Here's how the part is built. I have some questions about the finished solid (model axes, mm). Round coordinates to 2 decimals unless told otherwise and drop trailing zeros. Order: outer loops, then holes, each group sorted by start corner. A loop starts at its lowest first (then second) coordinate and runs counter-clockwise, first axis right, second up.
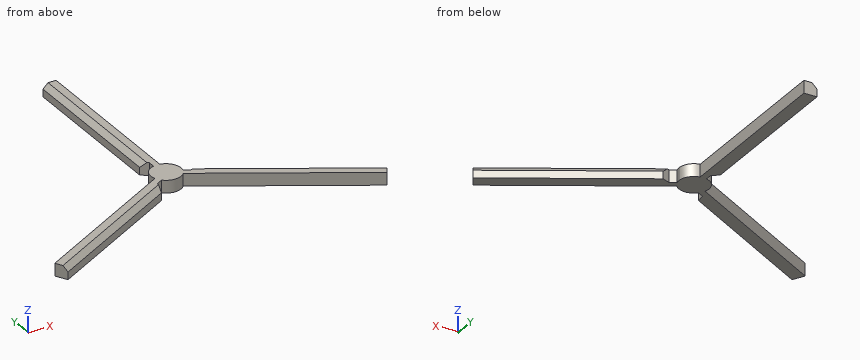
```python
from build123d import *

# Parameters (mm, degrees)
F1_DEPTH = 1.27
F2_SIZE  = 0.508


with BuildPart() as f1:
    # F0 (on Top) → F1 (new body)
    with BuildSketch(Plane.XY):
        with BuildLine():
            ThreePointArc((1.470624, -0.3998), (1.510597, -0.201674), (1.524, 0))
            ThreePointArc((1.524, 0), (1.166482, 0.980762), (0.261671, 1.501367))
            ThreePointArc((0.261671, 1.501367), (-0.065208, 1.522604), (-0.389075, 1.473498))
            ThreePointArc((-0.389075, 1.473498), (-1.351218, 0.70483), (-1.431058, -0.52407))
            ThreePointArc((-1.431058, -0.52407), (-1.28601, -0.817774), (-1.081549, -1.073698))
            ThreePointArc((-1.081549, -1.073698), (0.065208, -1.522604), (1.169387, -0.977297))
            ThreePointArc((1.169387, -0.977297), (1.351218, -0.70483), (1.470624, -0.3998))
        make_face()
        with BuildLine():
            ThreePointArc((-0.389075, 1.473498), (-0.065208, 1.522604), (0.261671, 1.501367))
            Line((0.261671, 1.501367), (0.261671, 19.281367))
            Line((0.261671, 19.281367), (-1.068548, 19.281367))
            Line((-1.068548, 19.281367), (-1.068548, 2.698131))
            Line((-1.068548, 2.698131), (-0.389075, 2.191366))
            Line((-0.389075, 2.191366), (-0.389075, 1.473498))
        make_face()
        with BuildLine():
            Line((2.092316, -0.758734), (1.470624, -0.3998))
            ThreePointArc((1.470624, -0.3998), (1.351218, -0.70483), (1.169387, -0.977297))
            Line((1.169387, -0.977297), (16.567319, -9.867297))
            Line((16.567319, -9.867297), (17.232428, -8.715294))
            Line((17.232428, -8.715294), (2.870924, -0.423675))
            Line((2.870924, -0.423675), (2.092316, -0.758734))
        make_face()
        with BuildLine():
            ThreePointArc((-1.081549, -1.073698), (-1.28601, -0.817774), (-1.431058, -0.52407))
            Line((-1.431058, -0.52407), (-16.82899, -9.41407))
            Line((-16.82899, -9.41407), (-16.16388, -10.566074))
            Line((-16.16388, -10.566074), (-1.802376, -2.274455))
            Line((-1.802376, -2.274455), (-1.703241, -1.432632))
            Line((-1.703241, -1.432632), (-1.081549, -1.073698))
        make_face()
    extrude(amount=F1_DEPTH)

    # F2
    f2_edges = [f1.edges().sort_by_distance(p)[0] for p in [
        (-1.068548, 10.989749, 1.27),
        (-8.983128, -6.420265, 1.27),
        (10.051676, -4.569485, 1.27),
    ]]
    chamfer(f2_edges, length=F2_SIZE)


solid = f1.part
```
1) If we section it at B-B (z = 0.2): Write out the boundary of the cut face in (x, y), plus the area to 3 significant figures.
2) If we section it at D-D (x = 11): Write out the boundary of the cut face in (y, z).
3) If we section it at A-A (y = -3.5): Write out the boundary of the cut face in (x, z).
4) I need wall thicknesses on line 1 (X direction, y = 13.5, z = 0.25); line 2 (X direction, y = -4.25, z = 0.35); line 3 (X direction, y = 7.5, z = 0.85). Which ranges of each line are inside material? Lowest first, please.
5) If we section it at C-C (y = 13.25): Write out the boundary of the cut face in (x, z), plus the area to 3 significant figures.
Solutions:
1. outline: (-16.83, -9.41) - (-16.16, -10.57) - (-1.8, -2.27) - (-1.7, -1.43) - (-1.08, -1.07) arc R1.52 ccw to (1.17, -0.98) - (16.57, -9.87) - (17.23, -8.72) - (2.87, -0.42) - (2.09, -0.76) - (1.47, -0.4) arc R1.52 ccw to (1.52, 0) arc R1.52 ccw to (0.26, 1.5) - (0.26, 19.28) - (-1.07, 19.28) - (-1.07, 2.7) - (-0.39, 2.19) - (-0.39, 1.47) arc R1.52 ccw to (-1.43, -0.52) - close
1. area: 76.3 mm2
2. outline: (-6.65, 0) - (-5.12, 0) - (-5.12, 0.76) - (-5.7, 1.27) - (-6.65, 1.27) - close
3. outline: (-6.59, 0) - (-3.93, 0) - (-3.93, 0.76) - (-4.94, 1.27) - (-6.59, 1.27) - close; (5.54, 0) - (8.2, 0) - (8.2, 0.76) - (7.18, 1.27) - (5.54, 1.27) - close
4. line 1: x = -1.07 to 0.26
4. line 2: x = -7.88 to -5.22, 6.84 to 9.5
4. line 3: x = -0.98 to 0.26
5. outline: (-1.07, 0) - (0.26, 0) - (0.26, 1.27) - (-0.56, 1.27) - (-1.07, 0.76) - close
5. area: 1.56 mm2
